The model under review builds one solid part; all positions refer to its coordinate system, in mm. Give positions to 0.01 mm unless a question says otherwise; leave off trailing zeros. Loops run counter-clockwise (first coordinate to the right, second up) from the corner with the lowest first, then second, coordinate; pieces in that order, holes last. Notation, with made-up numbers: (31, 1) - (74, 1) arc R33 ccw to (74, 34) - close; hole circle Ø6 at (79.5, -36). An arc over 180 degrees is marked (long way). Answer as a JSON object with one key per item and string values.
from build123d import *

# Parameters (mm, degrees)
F2_R     = 24.892
F5_DEPTH = 0.5
F1_W     = 5
F1_H     = 10
F6_DEPTH = 2.6162


# Not quite as in the source:
# - the program builds the solid bodies; features that only make, move or delete a surface that nothing else refers to are left out


with BuildPart() as f5:
    # F2 (on Front) → F5 (new body)
    with BuildSketch(Plane.XZ):
        Circle(F2_R)
    extrude(amount=F5_DEPTH)

    # F1 (on Front) → F6 (cut)
    with BuildSketch(Plane.XZ):
        with Locations((0, 18.4979066253)):
            Rectangle(F1_W, F1_H)
    extrude(amount=F6_DEPTH, mode=Mode.SUBTRACT)


solid = f5.part
Q1. Consider section D-D, the plane x = 18.5. State the section outline as (y, z) points, plus the area to 3 significant figures.
Results:
{"outline": "(-0.5, -16.65) - (0, -16.65) - (0, 16.65) - (-0.5, 16.65) - close", "area": "16.7 mm^2"}
Q2. To check wall thickness, follow probe 1 along Z at (x, y) = (-1.5, -0.05); probe 2 along X at (y, z) = (-0.3, 17.5); probe 3 along Z at (x, y) = (-3.5, -0.1). State the ranges of each line that lie inside material, in increasing order. Write a range as [from, to].
Results:
{"probe 1": "z = [-24.85, 13.5], [23.5, 24.85]", "probe 2": "x = [-17.7, -2.5], [2.5, 17.7]", "probe 3": "z = [-24.64, 24.64]"}
Q3. Clearance check with a flat-ended pin moving along its axis: pin 1 Ø1.5 at (x, z) = (-6, 10.5) entering from +Y. State where the tip first meets the part, or that it passes through.
Results:
{"pin 1": "stops at y = 0"}
Q4. Consider section A-A, the plane x = 0. State the section outline as (y, z) points, plus the area to 3 significant figures.
Results:
{"outline": "(-0.5, -24.89) - (0, -24.89) - (0, 13.5) - (-0.5, 13.5) - close; (-0.5, 23.5) - (0, 23.5) - (0, 24.89) - (-0.5, 24.89) - close", "area": "19.9 mm^2"}
Q5. Consider section B-B, the plane y = -0.25. State the section outline as (x, z) points, plus the area to 3 significant figures.
Results:
{"outline": "circle Ø49.78 at (0, 0); hole (-2.5, 13.5) - (2.5, 13.5) - (2.5, 23.5) - (-2.5, 23.5) - close", "area": "1,900 mm^2"}
Q6. Consider section C-C, the plane z = 15. State the section outline as (x, y) points, plus the area to 3 significant figures.
Results:
{"outline": "(-19.86, -0.5) - (-2.5, -0.5) - (-2.5, 0) - (-19.86, 0) - close; (2.5, -0.5) - (19.86, -0.5) - (19.86, 0) - (2.5, 0) - close", "area": "17.4 mm^2"}
